Geometry check sheet. Reference: the model listing, model coordinates, mm. A direction names the side the tool comes from. Coordinates: 2 decimals unless noted, no trailing zeros. Write each loop counter-clockwise with the first axis right and the second up, starting at its lowest first coordinate (ties: lowest second). Pieces come first, ordered by that corner, then holes.
from build123d import *

# Parameters (mm, degrees)
SKETCH_1_W      = 10
SKETCH_1_H      = 15
EXTRUDE_1_DEPTH = 10
EXTRUDE_2_DEPTH = 20
FILLET_1_R      = 5
FILLET_2_R      = 10


with BuildPart() as part:
    # 草圖1 → 填料-伸長1 (new body)
    with BuildSketch(Plane(origin=(0, 0, 0), x_dir=(1, 0, 0), z_dir=(0, 1, 0))):
        with Locations((5, -7.5)):
            Rectangle(SKETCH_1_W, SKETCH_1_H)
    extrude(amount=EXTRUDE_1_DEPTH)

    # 草圖1<3> → 填料-伸長2 (add)
    with BuildSketch(Plane(origin=(0, 0, 0), x_dir=(1, 0, 0), z_dir=(0, 1, 0))):
        Polygon((0, 10), (0, 0), (10, 0), (20, 0), (20, 10), align=None)
    extrude(amount=EXTRUDE_2_DEPTH)

    # 圓角1
    fillet_1_edges = [part.edges().sort_by_distance(p)[0] for p in [
        (5, 10, 15),
        (5, 10, 0),
    ]]
    fillet(fillet_1_edges, radius=FILLET_1_R)

    # 圓角2
    fillet_2_edges = [part.edges().sort_by_distance(p)[0] for p in [
        (20, 20, -5),
    ]]
    fillet(fillet_2_edges, radius=FILLET_2_R)


solid = part.part
1. Sectioned sample at A-A, the plane x = 3.25. Record the boundary of the cut face in (y, z), and give its area (3 significant figures).
Computed values:
outline: (0, -10) - (20, -10) - (20, 0) - (15, 0) arc R5 cw to (10, 5) - (10, 10) arc R5 ccw to (5, 15) - (0, 15) - close
area: 350 mm2
2. Gauge pin test, flat ends, axial feed: pin 1 Ø1.5 at (x, z) = (3, 6.5) entering from +Y; pin 2 Ø10 at (x, y) = (15.5, 14.5) entering from +Z; pin 3 Ø10 at (y, z) = (17, 6.5) entering from -X; pin 4 Ø7.5 at (y, z) = (5, 9.5) entering from +X. Record the tip position at first contact, or that the pin passes through.
Computed values:
pin 1: stops at y = 10
pin 2: stops at z = 0
pin 3: passes through
pin 4: stops at x = 10
3. Thickness scan on line 1 along X through (y, z) = (8, 13.5); line 2 along Z through (x, y) = (19, 1). Record the ranges inside material, lowest first.
Computed values:
line 1: x = 0 to 10
line 2: z = -10 to 0
4. Sectioned sample at D-D, the plane z = 13. Record the boundary of the cut face in (x, y), and give its area (3 significant figures).
Computed values:
outline: (0, 0) - (10, 0) - (10, 9) - (0, 9) - close
area: 90.0 mm2
5. Draft check along Y on faces 1 (the flat face through (12, 12, 0)), 2 (the flat face through (8, 0, 0)), 3 (the flat face through (5, 20, -5)). Enter one of: released by +Y, released by -Y, zero draft, split by the parting line, or undercut.
Computed values:
face 1: zero draft
face 2: released by -Y
face 3: released by +Y
6. Sectioned sample at B-B, the plane y = 2.25. Record the boundary of the cut face in (x, z).
Computed values:
outline: (0, -10) - (20, -10) - (20, 0) - (10, 0) - (10, 15) - (0, 15) - close
7. Sectioned sample at C-C, the plane z = -3.5. Record the boundary of the cut face in (x, y), and give its area (3 significant figures).
Computed values:
outline: (0, 0) - (20, 0) - (20, 10) arc R10 ccw to (10, 20) - (0, 20) - close
area: 379 mm2
8. Access from +Z, -Z, +X, -X, +Y, -Y to the whole of each face (thin tool, end or side, straight path). Record for faces 4 (the flat face through (10, 6, 8)), 5 (the flat face through (10, 10, -10)), 6 (the flat face through (5, 10, 7)).
Computed values:
face 4: +Z, +X, +Y, -Y
face 5: -Z, +X, -X, +Y, -Y
face 6: +Z, +X, -X, +Y
